from build123d import *

# Parameters (mm, degrees)
MODEL_W                  = 79.9
MODEL_H                  = 102.298269881
MODEL_R                  = 1.8
MODEL_W_2                = 6.8
MODEL_H_2                = 10.4
MODEL_W_3                = 6.9
MODEL_H_3                = 20.768459162
RESSALTO_EXTRUS_O1_DEPTH = 6


with BuildPart() as part:
    # Model → Ressalto-extrusão1 (new body)
    with BuildSketch(Plane.XY):
        with Locations((69.087325958, 59.378502518)):
            Rectangle(MODEL_W, MODEL_H)
        with Locations((52.637325958, 12.745101048)):
            Circle(MODEL_R, mode=Mode.SUBTRACT)
        with Locations((85.537325958, 12.745101048)):
            Circle(MODEL_R, mode=Mode.SUBTRACT)
        with Locations((91.587325958, 51.927637459)):
            Circle(MODEL_R, mode=Mode.SUBTRACT)
        with Locations((46.587325958, 51.927637459)):
            Circle(MODEL_R, mode=Mode.SUBTRACT)
        with Locations((99.037325958, 97.527637459)):
            Rectangle(MODEL_W_2, MODEL_H_2, mode=Mode.SUBTRACT)
        with Locations((39.137325958, 97.527637459)):
            Rectangle(MODEL_W_2, MODEL_H_2, mode=Mode.SUBTRACT)
        with Locations((99.037325958, 43.927637459)):
            Rectangle(MODEL_W_2, MODEL_H_2, mode=Mode.SUBTRACT)
        with Locations((39.137325958, 18.427637459)):
            Rectangle(MODEL_W_2, MODEL_H_2, mode=Mode.SUBTRACT)
        with Locations((53.787325958, 37.060868969)):
            Rectangle(MODEL_W_3, MODEL_H_3, mode=Mode.SUBTRACT)
        with BuildLine():
            Line((52.037325958, 70.571372091), (52.037325958, 64.371372091))
            ThreePointArc((52.037325958, 64.371372091), (53.637325958, 62.771372091), (55.237325958, 64.371372091))
            Line((55.237325958, 64.371372091), (55.237325958, 70.571372091))
            ThreePointArc((55.237325958, 70.571372091), (53.637325958, 72.171372091), (52.037325958, 70.571372091))
        make_face(mode=Mode.SUBTRACT)
        with Locations((84.387325958, 37.060868969)):
            Rectangle(MODEL_W_3, MODEL_H_3, mode=Mode.SUBTRACT)
        with Locations((99.037325958, 18.427637459)):
            Rectangle(MODEL_W_2, MODEL_H_2, mode=Mode.SUBTRACT)
        with BuildLine():
            Line((86.237325958, 70.571372091), (86.237325958, 64.371372091))
            ThreePointArc((86.237325958, 64.371372091), (84.637325958, 62.771372091), (83.037325958, 64.371372091))
            Line((83.037325958, 64.371372091), (83.037325958, 70.571372091))
            ThreePointArc((83.037325958, 70.571372091), (84.637325958, 72.171372091), (86.237325958, 70.571372091))
        make_face(mode=Mode.SUBTRACT)
        with BuildLine():
            Line((86.237325958, 101.571372091), (86.237325958, 95.371372091))
            ThreePointArc((86.237325958, 95.371372091), (84.637325958, 93.771372091), (83.037325958, 95.371372091))
            Line((83.037325958, 95.371372091), (83.037325958, 101.571372091))
            ThreePointArc((83.037325958, 101.571372091), (84.637325958, 103.171372091), (86.237325958, 101.571372091))
        make_face(mode=Mode.SUBTRACT)
        with Locations((39.137325958, 43.927637459)):
            Rectangle(MODEL_W_2, MODEL_H_2, mode=Mode.SUBTRACT)
        with BuildLine():
            Line((52.037325958, 101.571372091), (52.037325958, 95.371372091))
            ThreePointArc((52.037325958, 95.371372091), (53.637325958, 93.771372091), (55.237325958, 95.371372091))
            Line((55.237325958, 95.371372091), (55.237325958, 101.571372091))
            ThreePointArc((55.237325958, 101.571372091), (53.637325958, 103.171372091), (52.037325958, 101.571372091))
        make_face(mode=Mode.SUBTRACT)
        with BuildLine():
            Line((54.137325958, 86.071372091), (54.137325958, 79.871372091))
            ThreePointArc((54.137325958, 79.871372091), (69.137325958, 64.871372091), (84.137325958, 79.871372091))
            Line((84.137325958, 79.871372091), (84.137325958, 86.071372091))
            ThreePointArc((84.137325958, 86.071372091), (69.137325958, 101.071372091), (54.137325958, 86.071372091))
        make_face(mode=Mode.SUBTRACT)
    extrude(amount=RESSALTO_EXTRUS_O1_DEPTH)


solid = part.part
Geometry check sheet. Reference: the model listing, model coordinates, mm. A direction names the side the tool comes from. Give positions to 0.01 mm unless a question says otherwise; leave off trailing zeros. Write each loop counter-clockwise with the first axis right and the second up, starting at its lowest first coordinate (ties: lowest second). Pieces come first, ordered by that corner, then holes. Notation, with made-up numbers: (48.25, 88) - (96.25, 88) arc R23 cw to (96.25, 107) - close; hole circle Ø10 at (-28, -16). An arc over 180 degrees is marked (long way). Put each result on its own line as item: value.
1. Set-up check for faces 4 (the flat face through (86.237, 99, 3)), 5 (the flat face through (69, 60, 0)): record each of +Z, -Z, +X, -X, +Y, -Y from which the full face is reachable in a straight line by a thin tool's end or side.
Ans:
face 4: +Z, -Z
face 5: -Z, +X, -X, +Y, -Y
2. Sectioned sample at A-A, the plane y = 46. Enter the section's corners in (x, z).
Ans:
outline: (29.14, 0) - (35.74, 0) - (35.74, 6) - (29.14, 6) - close; (42.54, 0) - (50.34, 0) - (50.34, 6) - (42.54, 6) - close; (57.24, 0) - (80.94, 0) - (80.94, 6) - (57.24, 6) - close; (87.84, 0) - (95.64, 0) - (95.64, 6) - (87.84, 6) - close; (102.44, 0) - (109.04, 0) - (109.04, 6) - (102.44, 6) - close
3. Draft check along Y on faces 1 (the flat face through (54, 26.677, 3)), 2 (the flat face through (69, 60, 6)), 3 (the cylindrical face through (53.67, 103.17, 2.96)). Enter one of: +Y half, -Y half, draft (parallel to the pull), parting line (faces both ways), or undercut.
Ans:
face 1: undercut
face 2: draft
face 3: undercut
4. Go/stop test with a flat-tipped pin: pin 1 (3 mm diameter, centred on x = 52.64, y = 12.75, fed in from -Z). Record where the tip stops, or that it passes through.
Ans:
pin 1: passes through
5. Sectioned sample at D-D, the plane z = 3.1. Give the number of separate pieces and of enclosed holes in the cut face, plus the area to 3 significant figures.
Ans:
separate pieces: 1
enclosed holes: 17
area: 6,420 mm²
6. Sectioned sample at C-C, the plane x = 69. Enter the section's corners in (y, z), plus the area to 3 significant figures.
Ans:
outline: (8.23, 0) - (64.87, 0) - (64.87, 6) - (8.23, 6) - close; (101.07, 0) - (110.53, 0) - (110.53, 6) - (101.07, 6) - close
area: 397 mm²
7. Thickness scan on line 1 (X direction, y = 17, z = 0.5); line 2 (X direction, y = 27, z = 0.4); line 3 (Y direction, x = 37.5, z = 2.8). Record the ranges inside material, lowest first.
Ans:
line 1: x = 29.14 to 35.74, 42.54 to 95.64, 102.44 to 109.04
line 2: x = 29.14 to 50.34, 57.24 to 80.94, 87.84 to 109.04
line 3: y = 8.23 to 13.23, 23.63 to 38.73, 49.13 to 92.33, 102.73 to 110.53
8. Sectioned sample at B-B, the plane x = 98. Enter the section's corners in (y, z).
Ans:
outline: (8.23, 0) - (13.23, 0) - (13.23, 6) - (8.23, 6) - close; (23.63, 0) - (38.73, 0) - (38.73, 6) - (23.63, 6) - close; (49.13, 0) - (92.33, 0) - (92.33, 6) - (49.13, 6) - close; (102.73, 0) - (110.53, 0) - (110.53, 6) - (102.73, 6) - close
